```python
from build123d import *

# Parameters (mm, degrees)
F0_W     = 25.4
F0_H     = 6.35
F1_DEPTH = 6.35


with BuildPart() as f1:
    # F0 (on Top) → F1 (new body)
    with BuildSketch(Plane.XY):
        Polygon((-171.779727, 16), (-171.779727, 0), (-146.379727, 0), (-120.979727, 0), (-12.7, 0), (12.7, 0), (120.979727, 0), (146.379727, 0), (171.779727, 0), (171.779727, 16), (127.261273, 10.935512), (102.024054, 8.064488), (57.5056, 3), (12.7, 3), (-12.7, 3), (-57.5056, 3), (-102.024054, 8.064488), (-127.261273, 10.935512), align=None)
        with Locations((-133.679727, -3.175)):
            Rectangle(F0_W, F0_H)
        Polygon((-126.543517, 17.244817), (-127.261273, 10.935512), (-102.024054, 8.064488), (-101.306298, 14.373792), align=None)
        with Locations((0, -3.175)):
            Rectangle(F0_W, F0_H)
        with Locations((133.679727, -3.175)):
            Rectangle(F0_W, F0_H)
        with Locations((0, 6.175)):
            Rectangle(F0_W, F0_H)
        Polygon((101.306298, 14.373792), (102.024054, 8.064488), (127.261273, 10.935512), (126.543517, 17.244817), align=None)
    extrude(amount=F1_DEPTH)


solid = f1.part
```
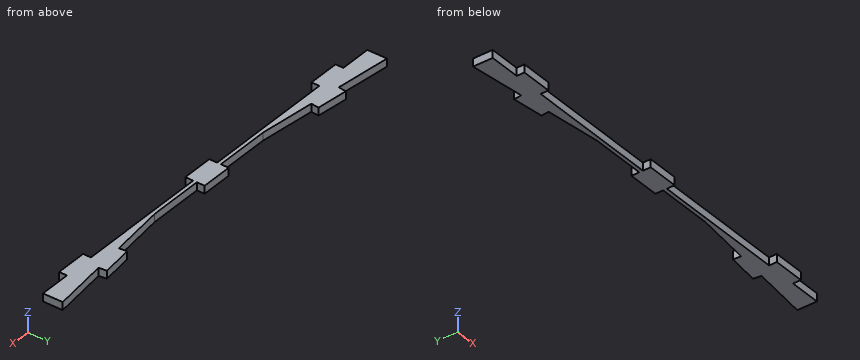
Source: CAD feature listing. Evaluate the final solid. Frame: model axes, mm. Round coordinates to 2 decimals unless told otherwise and drop trailing zeros. Order: outer loops, then holes, each group sorted by start corner. A loop starts at its lowest first (then second) coordinate and runs counter-clockwise, first axis right, second up. Notation, with made-up numbers: (47, -23.5) -> (64, -23.5) arc R7 ccw to (64, -15.5) -> close; hole circle Ø11 at (22.5, 50). An arc over 180 degrees is marked (long way). One line per item, written item: value. Start each with the question number.
Q1. Section query D-D (x = -7). Return the cut outline in (y, z).
Q2. Section query C-C (x = -131). Return the cut outline in (y, z), plus the area to 3 significant figures.
Q3. Pin query (flat end, axial travel): pin 1 (3 mm diameter, centred on x = -2, z = 2, fed in from +Y); pin 2 (2 mm diameter, centred on x = -115.5, y = -2.5, fed in from -Z); pin 3 (3 mm diameter, centred on x = -46, z = 4.5, fed in from +Y); pin 4 (1.9 mm diameter, centred on x = 79.5, z = 4, fed in from -Y). Return the tip coordinate at first contact, or that it passes through.
Q4. Section query A-A (y = -3). Return the cut outline in (x, z), plus the area to 3 significant figures.
Q5. Material intervals for probe 1 along X at (y, z) = (-4.5, 4.25); probe 2 along X at (y, z) = (9.25, 4); probe 3 along Y at (x, z) = (-8.5, 2.25), sorted ascending.
Findings below:
1. outline: (-6.35, 0) -> (9.35, 0) -> (9.35, 6.35) -> (-6.35, 6.35) -> close
2. outline: (-6.35, 0) -> (11.36, 0) -> (11.36, 6.35) -> (-6.35, 6.35) -> close
2. area: 112 mm²
3. pin 1: y = 9.35
3. pin 2: through
3. pin 3: y = 3
3. pin 4: y = 0
4. outline: (-146.38, 0) -> (-120.98, 0) -> (-120.98, 6.35) -> (-146.38, 6.35) -> close; (-12.7, 0) -> (12.7, 0) -> (12.7, 6.35) -> (-12.7, 6.35) -> close; (120.98, 0) -> (146.38, 0) -> (146.38, 6.35) -> (120.98, 6.35) -> close
4. area: 484 mm²
5. probe 1: -146.38 to -120.98, -12.7 to 12.7, 120.98 to 146.38
5. probe 2: -171.78 to -101.89, -12.7 to 12.7, 101.89 to 171.78
5. probe 3: -6.35 to 9.35
